Can you work these out from the model? Positions are in its coordinate system, mm. A direction names the side the tool comes from. Coordinates: 2 decimals unless noted, no trailing zeros. Order: outer loops, then holes, each group sorted by start corner. A loop starts at its lowest first (then second) coordinate and runs counter-clockwise, first axis right, second up. Notation, with made-up numbers: (-5, 34) -> (6, 34) arc R13 cw to (6, 57) -> close; hole circle Ø5 at (7, 62.5). An arc over 180 degrees is marked (long way). Answer as a JSON object with one key per item and string values. Group by question number.
(1) I want a section at B-B, the plane z = -14.5. List the corners of the cut face in (x, y) for me, plus the area to 3 significant figures.
(2) If we mould it in two halves opening along Y, with no side actions, what happens to faces 4 (the conical face through (80.3, 31.8, -15.3)), 5 (the cylindrical face through (61.776, 37.534, -10.232)), 6 (the flat face through (66, 39, -11.5)), 7 (the conical face through (80.82, 43.64, -8.64))? For each: pulls with the +Y half, pulls with the -Y half, needs draft (parallel to the pull), parting line crosses it, or undercut.
(3) I need wall thicknesses on line 1 (Z direction, x = 66.5, y = 35); line 2 (X direction, y = 35, z = -15); line 3 (X direction, y = 37.25, z = -14). Which ranges of each line are inside material? Lowest first, please.
(4) For pin 1 (8 mm diameter, centred on x = 72.5, y = 35.5, fed in from -Z); pin 2 (2 mm diameter, centred on x = 86.5, y = 38.5, fed in from -Z); pin 3 (2 mm diameter, centred on x = 65.5, y = 36.5, fed in from +Z); pin 4 (1.6 mm diameter, centred on x = 78.5, z = -10, fed in from +Y), each with a flat end and sliding along its axis, tell me the tip position at first contact or that it passes through.
(5) Which directions (+Z, -Z, +X, -X, +Y, -Y) give clear straight access to the entire face, cutting with the end or side of a thin tool? Please do faces 1 (the flat face through (81, 38, -10.5)), 2 (the cylindrical face through (86.923, 40.973, -15.021)), 3 (the cylindrical face through (80.3, 31.5, -12)).
(6) I want a section at A-A, the plane z = -12. List the corners of the cut face in (x, y) for me, plus the area to 3 significant figures.
from build123d import *

# Parameters (mm, degrees)
EXTRUDE_1_DEPTH              = 8
CHAMFER_7_SIZE               = 1.5
HOLE_WIZARD_M3_1_D           = 3.2
HOLE_WIZARD_M3_1_CBORE_D     = 6.5
HOLE_WIZARD_M3_1_CBORE_DEPTH = 3
HOLE_WIZARD_M3_2_D           = 3.2
HOLE_WIZARD_M3_2_CBORE_D     = 6.5
HOLE_WIZARD_M3_2_CBORE_DEPTH = 3
CUT_EXTRUDE_6_DEPTH          = 2
CHAMFER_8_SIZE               = 0.5
CHAMFER_9_SIZE               = 0.5


with BuildPart() as part:
    # ｽｹｯﾁ3 → ﾎﾞｽ - 押し出し1 (new body)
    with BuildSketch(Plane.XY.offset(-16.5)):
        with BuildLine():
            Line((58.49999999, 38.105482977), (64.74999999, 27.280165429))
            ThreePointArc((64.74999999, 27.280165429), (80.49999999, 31.50036521), (96.24999999, 27.280165429))
            Line((96.24999999, 27.280165429), (102.49999999, 38.105482977))
            ThreePointArc((102.49999999, 38.105482977), (80.49999999, 44.00036521), (58.49999999, 38.105482977))
        make_face()
    extrude(amount=EXTRUDE_1_DEPTH)

    # 面取り7
    chamfer_7_edges = [part.edges().sort_by_distance(p)[0] for p in [
        (80.49999999, 31.50036521, -16.5),
    ]]
    chamfer(chamfer_7_edges, length=CHAMFER_7_SIZE)

    # M3 穴付きねじ用座ぐり穴1 (through all)
    with Locations(Plane.XY.offset(-8.5)):
        with Locations((65.0229264, 37.390950693), (95.977073581, 37.390950693)):
            CounterBoreHole(HOLE_WIZARD_M3_1_D / 2, HOLE_WIZARD_M3_1_CBORE_D / 2, HOLE_WIZARD_M3_1_CBORE_DEPTH)

    # M3 穴付きねじ用座ぐり穴2 (through all)
    with Locations(Plane(origin=(0, 0, -16.5), x_dir=(-1, 0, 0), z_dir=(0, 0, -1))):
        with Locations((-86.49999999, 37.75036521), (-74.49999999, 37.75036521)):
            CounterBoreHole(HOLE_WIZARD_M3_2_D / 2, HOLE_WIZARD_M3_2_CBORE_D / 2, HOLE_WIZARD_M3_2_CBORE_DEPTH)

    # ｽｹｯﾁ17 → ｶｯﾄ - 押し出し6 (cut)
    with BuildSketch(Plane.XY.offset(-8.5)):
        with BuildLine():
            Line((73.49999999, 41.75036521), (87.49999999, 41.75036521))
            ThreePointArc((87.49999999, 41.75036521), (89.621320334, 40.871685554), (90.49999999, 38.75036521))
            Line((90.49999999, 38.75036521), (90.49999999, 36.75036521))
            ThreePointArc((90.49999999, 36.75036521), (89.621320334, 34.629044867), (87.49999999, 33.75036521))
            Line((87.49999999, 33.75036521), (73.49999999, 33.75036521))
            ThreePointArc((73.49999999, 33.75036521), (71.378679647, 34.629044867), (70.49999999, 36.75036521))
            Line((70.49999999, 36.75036521), (70.49999999, 38.75036521))
            ThreePointArc((70.49999999, 38.75036521), (71.378679647, 40.871685554), (73.49999999, 41.75036521))
        make_face()
    extrude(amount=-CUT_EXTRUDE_6_DEPTH, mode=Mode.SUBTRACT)

    # 面取り8
    # the kernel refuses this chamfer: 0.5 mm, written as the material it takes off along each edge
    with BuildSketch(Plane(origin=(80.49999999, 0.00036521, -8.5), x_dir=(-0.5349312949950591, 0.844895561377209, 0), z_dir=(-0.844895561377209, -0.5349312949950591, 0))) as chamfer_8_piece_1:
        Polygon((31.5, CHAMFER_8_SIZE), (31.5 + CHAMFER_8_SIZE, 0), (31.5, 0), align=None)
    revolve(axis=Axis((80.49999999, 0.00036521, -8.5), (0, 0, -1)), revolution_arc=64.678504259, mode=Mode.SUBTRACT)
    with BuildSketch(Plane(origin=(95.607079243, 26.16659403, -8.5), x_dir=(-0.8660254037844379, 0.5000000000000012, 0), z_dir=(0.5000000000000012, 0.866025403784438, 0))) as chamfer_8_piece_2:
        Polygon((CHAMFER_8_SIZE, 0), (0, -CHAMFER_8_SIZE), (0, 0), align=None)
    extrude(amount=15.071682988, mode=Mode.SUBTRACT)
    with BuildSketch(Plane(origin=(80.49999999, 0.00036521, -8.5), x_dir=(0.5250957878127545, 0.8510431326444641, 0), z_dir=(0.8510431326444641, -0.5250957878127545, 0))) as chamfer_8_piece_3:
        Polygon((44 - CHAMFER_8_SIZE, 0), (44, -CHAMFER_8_SIZE), (44, 0), align=None)
    revolve(axis=Axis((80.49999999, 0.00036521, -8.5), (0, 0, 1)), revolution_arc=63.349383731, mode=Mode.SUBTRACT)
    with BuildSketch(Plane(origin=(95.977073581, 37.390950693, -8.5), x_dir=(1, 0, 0), z_dir=(0, -1, 0))) as chamfer_8_piece_4:
        Polygon((3.25 + CHAMFER_8_SIZE, 0), (3.25, -CHAMFER_8_SIZE), (3.25, 0), align=None)
    revolve(axis=Axis((95.977073581, 37.390950693, -8.5), (0, 0, 1)), mode=Mode.SUBTRACT)
    with BuildSketch(Plane(origin=(65.0229264, 37.390950693, -8.5), x_dir=(1, 0, 0), z_dir=(0, -1, 0))) as chamfer_8_piece_5:
        Polygon((3.25 + CHAMFER_8_SIZE, 0), (3.25, -CHAMFER_8_SIZE), (3.25, 0), align=None)
    revolve(axis=Axis((65.0229264, 37.390950693, -8.5), (0, 0, 1)), mode=Mode.SUBTRACT)
    with BuildSketch(Plane(origin=(57.857079243, 39.219054376, -8.5), x_dir=(0, 0, -1), z_dir=(0.5000000000000007, -0.8660254037844384, 0))) as chamfer_8_piece_6:
        Polygon((CHAMFER_8_SIZE, 0), (0, CHAMFER_8_SIZE), (0, 0), align=None)
    extrude(amount=15.071682988, mode=Mode.SUBTRACT)
    with BuildSketch(Plane(origin=(87.49999999, 38.75036521, -8.5), x_dir=(0, 1, 0), z_dir=(-1, 0, 0))) as chamfer_8_piece_7:
        Polygon((3 + CHAMFER_8_SIZE, 0), (3, CHAMFER_8_SIZE), (3, 0), align=None)
    revolve(axis=Axis((87.49999999, 38.75036521, -8.5), (0, 0, -1)), revolution_arc=90, mode=Mode.SUBTRACT)
    with BuildSketch(Plane(origin=(73.49999999, 41.75036521, -8.5), x_dir=(0, 1, 0), z_dir=(1, 0, 0)), Plane(origin=(87.49999999, 33.75036521, -8.5), x_dir=(0, -1, 0), z_dir=(-1, 0, 0))) as chamfer_8_piece_8:
        Polygon((CHAMFER_8_SIZE, 0), (0, -CHAMFER_8_SIZE), (0, 0), align=None)
    extrude(amount=14, mode=Mode.SUBTRACT)
    with BuildSketch(Plane(origin=(73.49999999, 38.75036521, -8.5), x_dir=(-1, 0, 0), z_dir=(0, -1, 0))) as chamfer_8_piece_9:
        Polygon((3 + CHAMFER_8_SIZE, 0), (3, CHAMFER_8_SIZE), (3, 0), align=None)
    revolve(axis=Axis((73.49999999, 38.75036521, -8.5), (0, 0, -1)), revolution_arc=90, mode=Mode.SUBTRACT)
    with BuildSketch(Plane(origin=(70.49999999, 36.75036521, -8.5), x_dir=(-1, 0, 0), z_dir=(0, 1, 0)), Plane(origin=(90.49999999, 38.75036521, -8.5), x_dir=(1, 0, 0), z_dir=(0, -1, 0))) as chamfer_8_piece_10:
        Polygon((CHAMFER_8_SIZE, 0), (0, -CHAMFER_8_SIZE), (0, 0), align=None)
    extrude(amount=2, mode=Mode.SUBTRACT)
    with BuildSketch(Plane(origin=(73.49999999, 36.75036521, -8.5), x_dir=(0, -1, 0), z_dir=(1, 0, 0))) as chamfer_8_piece_11:
        Polygon((3 + CHAMFER_8_SIZE, 0), (3, CHAMFER_8_SIZE), (3, 0), align=None)
    revolve(axis=Axis((73.49999999, 36.75036521, -8.5), (0, 0, -1)), revolution_arc=90, mode=Mode.SUBTRACT)
    with BuildSketch(Plane(origin=(87.49999999, 36.75036521, -8.5), x_dir=(1, 0, 0), z_dir=(0, 1, 0))) as chamfer_8_piece_12:
        Polygon((3 + CHAMFER_8_SIZE, 0), (3, CHAMFER_8_SIZE), (3, 0), align=None)
    revolve(axis=Axis((87.49999999, 36.75036521, -8.5), (0, 0, -1)), revolution_arc=90, mode=Mode.SUBTRACT)

    # 面取り9
    # the kernel refuses this chamfer: 0.5 mm, written as the material it takes off along each edge
    with BuildSketch(Plane(origin=(96.24999999, 27.280165429, -16.296233904), x_dir=(-0.8699980733677616, 0.4930551209919465, 0), z_dir=(0, 0, 1))) as chamfer_9_piece_1:
        with BuildLine():
            Line((0.504048916, 0), (-CHAMFER_9_SIZE * 0.00800077643885, -CHAMFER_9_SIZE * 0.999967993276))
            Line((-CHAMFER_9_SIZE * 0.00800077643885, -CHAMFER_9_SIZE * 0.999967993276), (0, 0))
            ThreePointArc((0, 0), (0.259153689, -0.001007405), (0.504048916, 0))
        make_face()
    extrude(amount=8.592467809, mode=Mode.SUBTRACT)
    with BuildSketch(Plane(origin=(64.74999999, 27.280165429, -16.296233904), x_dir=(-0.499999999999999, 0.8660254037844393, 0), z_dir=(0, 0, 1))) as chamfer_9_piece_2:
        with BuildLine():
            Line((CHAMFER_9_SIZE, 0), (-0.004032783, -0.504032783))
            ThreePointArc((-0.004032783, -0.504032783), (-0.001066058, -0.259153454), (0, 0))
            Line((0, 0), (CHAMFER_9_SIZE, 0))
        make_face()
    extrude(amount=8.592467809, mode=Mode.SUBTRACT)
    with BuildSketch(Plane(origin=(58.49999999, 38.105482977, -17.785841494), x_dir=(0.5000000000000021, -0.8660254037844375, 0), z_dir=(0, 0, 1))) as chamfer_9_piece_3:
        with BuildLine():
            Line((CHAMFER_9_SIZE, 0), (0.002809166, 0.497190834))
            ThreePointArc((0.002809166, 0.497190834), (0.000742578, 0.255629249), (0, 0))
            Line((0, 0), (CHAMFER_9_SIZE, 0))
        make_face()
    extrude(amount=10.071682988, mode=Mode.SUBTRACT)
    with BuildSketch(Plane(origin=(102.49999999, 38.105482977, -17.785841494), x_dir=(-0.8688365739050292, 0.4950989879256175, 0), z_dir=(0, 0, 1))) as chamfer_9_piece_4:
        with BuildLine():
            Line((0.49719877, 0), (CHAMFER_9_SIZE * 0.00564998602096, CHAMFER_9_SIZE * 0.999984038702))
            Line((CHAMFER_9_SIZE * 0.00564998602096, CHAMFER_9_SIZE * 0.999984038702), (0, 0))
            ThreePointArc((0, 0), (0.255629364, -0.000701736), (0.49719877, 0))
        make_face()
    extrude(amount=10.071682988, mode=Mode.SUBTRACT)


solid = part.part
Computed values:
{
 "1": {"outline": "(58.75, 37.67) -> (64.5, 27.71) -> (65.19, 27.53) arc R31.5 cw to (95.81, 27.53) -> (96.5, 27.71) -> (102.25, 37.67) -> (102.07, 38.35) arc R44 ccw to (58.93, 38.35) -> close; hole circle Ø3.2 at (65.02, 37.39); hole circle Ø6.5 at (74.5, 37.75); hole circle Ø6.5 at (86.5, 37.75); hole circle Ø3.2 at (95.98, 37.39)", "area": "411 mm2"},
 "2": {"face 4": "pulls with the -Y half", "face 5": "undercut", "face 6": "undercut", "face 7": "pulls with the +Y half"},
 "3": {"line 1": "z = -16.5 to -11.5", "line 2": "x = 60.29 to 72.77, 76.23 to 84.77, 88.23 to 100.71", "line 3": "x = 58.99 to 63.43, 66.62 to 71.29, 77.71 to 83.29, 89.71 to 94.38, 97.57 to 102.01"},
 "4": {"pin 1": "stops at z = -16.5", "pin 2": "stops at z = -13.5", "pin 3": "stops at z = -11.5", "pin 4": "stops at y = 43.98"},
 "5": {"face 1": "+Z", "face 2": "-Z", "face 3": "+Z, -Z, -Y"},
 "6": {"outline": "(58.75, 37.67) -> (64.5, 27.71) -> (65.19, 27.53) arc R31.5 cw to (95.81, 27.53) -> (96.5, 27.71) -> (102.25, 37.67) -> (102.07, 38.35) arc R44 ccw to (58.93, 38.35) -> close; hole circle Ø3.2 at (65.02, 37.39); hole circle Ø3.2 at (74.5, 37.75); hole circle Ø3.2 at (86.5, 37.75); hole circle Ø3.2 at (95.98, 37.39)", "area": "461 mm2"}
}
